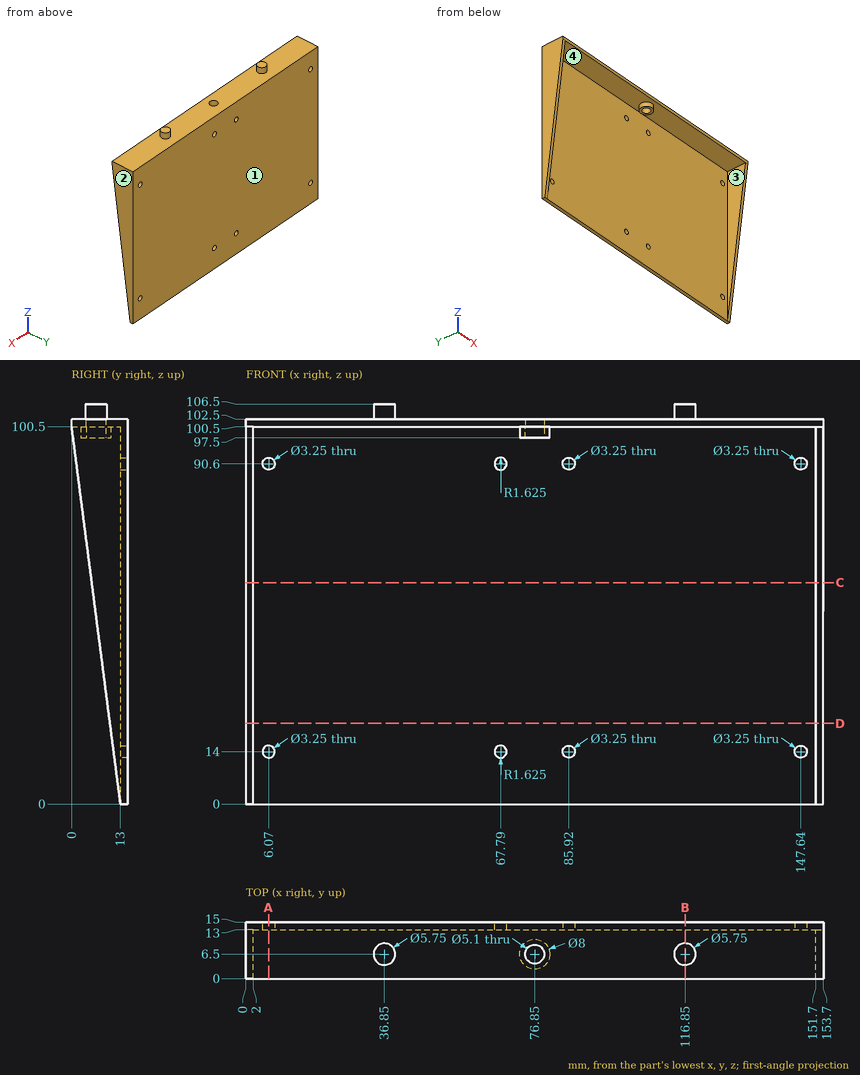
Study the drawing (mm; zero at the part's minimum x, y, z) and answer. Give positions to 0.01 mm unless a question says otherwise; leave off trailing zeros. Write each loop counter-clockwise with the first axis right and the second up, starting at its lowest first coordinate (ties: lowest second). Pieces come first, ordered by that corner, then holes.
(1) Flat-ended cylindrical pins translate along their axes: pin 1 Ø1.5 at (x, y) = (45.5, 7.5) entering from -Z; pin 2 Ø5 at (x, z) = (85.92, 90.6) entering from -Y; pin 3 Ø4 at (x, y) = (79, 7.5) entering from -Z. Find the tip coordinate at first contact, or state that the pin passes through.
Final values:
pin 1: stops at z = 100.5
pin 2: stops at y = 13
pin 3: stops at z = 97.5
(2) The part is cut by section D-D on z = 21.5. Write down the section's boundary in (x, y).
Final values:
outline: (0, 10.22) - (2, 10.22) - (2, 13) - (151.7, 13) - (151.7, 10.22) - (153.7, 10.22) - (153.7, 15) - (0, 15) - close
(3) The part is cut by section B-B on x = 116.85. Write down the section's boundary in (y, z) (3 decimals), plus the area to 3 significant figures.
Final values:
outline: (0, 100.5) - (13, 100.5) - (13, 0) - (15, 0) - (15, 102.5) - (9.375, 102.5) - (9.375, 106.5) - (3.625, 106.5) - (3.625, 102.5) - (0, 102.5) - close
area: 254 mm2
(4) The part is cut by section C-C on z = 59. Write down the section's boundary in (x, y), plus the area to 3 significant figures.
Final values:
outline: (0, 5.37) - (2, 5.37) - (2, 13) - (151.7, 13) - (151.7, 5.37) - (153.7, 5.37) - (153.7, 15) - (0, 15) - close
area: 338 mm2
(5) Straight lines are drawn through the part: line 1 (Z direction, x = 147.64, y = 14.4) (3 decimals); line 2 (X direction, y = 13.6, z = 90.6) (3 decimals); line 3 (X direction, y = 11.5, z = 82.5). For each, find the intervals that lie inside material, in ascending order.
Final values:
line 1: z = 0 to 12.375, 15.625 to 88.975, 92.225 to 102.5
line 2: x = 0 to 4.445, 7.695 to 66.165, 69.415 to 84.295, 87.545 to 146.015, 149.265 to 153.7
line 3: x = 0 to 2, 151.7 to 153.7
(6) The part is cut by section A-A on x = 6.07. Write down the section's boundary in (y, z) (3 decimals), plus the area to 3 significant figures.
Final values:
outline: (0, 100.5) - (13, 100.5) - (13, 92.225) - (15, 92.225) - (15, 102.5) - (0, 102.5) - close; (13, 0) - (15, 0) - (15, 12.375) - (13, 12.375) - close; (13, 15.625) - (15, 15.625) - (15, 88.975) - (13, 88.975) - close
area: 218 mm2
(7) The mould has two halves that part along X. Classify the marked faces 1, 2, 3 and 4: pulls with the +X half, pulls with the -X half, needs draft (parallel to the pull), parting line crosses it, or undercut.
Final values:
face 1: needs draft
face 2: pulls with the +X half
face 3: undercut
face 4: undercut
